```python
from build123d import *

# Parameters (mm, degrees)
BOSS_EXTRUDE1_DEPTH = 110


with BuildPart() as part:
    # Sketch1 → Boss-Extrude1 (new body)
    with BuildSketch(Plane.XY):
        Polygon((0, 12.5), (0, 0), (2, 0), (2, 9.5), (4, 9.5), (4, 0), (6, 0), (6, 9.5), (8, 9.5), (8, 0), (10, 0), (10, 9.5), (12, 9.5), (12, 0), (14, 0), (14, 9.5), (23.5, 9.5), (23.5, 12.5), align=None)
        Polygon((47, 12.5), (23.5, 12.5), (23.5, 9.5), (33, 9.5), (33, 0), (35, 0), (35, 9.5), (37, 9.5), (37, 0), (39, 0), (39, 9.5), (41, 9.5), (41, 0), (43, 0), (43, 9.5), (45, 9.5), (45, 0), (47, 0), align=None)
    extrude(amount=BOSS_EXTRUDE1_DEPTH)


solid = part.part
```
Geometry check sheet. Reference: the model listing, model coordinates, mm. A direction names the side the tool comes from. Coordinates: 2 decimals unless noted, no trailing zeros. Order: outer loops, then holes, each group sorted by start corner. A loop starts at its lowest first (then second) coordinate and runs counter-clockwise, first axis right, second up. Notation, with made-up numbers: M 34,-30 L 74,-30 A30 cw 74,-5 Z; hole C -0.5,7 d9. An arc over 180 degrees is marked long. Answer as a JSON object with one key per item and string values.
Q1. Tool access check on faces 1 (the flat face through (42, 0, 54)), 2 (the flat face through (45, 5, 54)). Record the directions out of +Z, -Z, +X, -X, +Y, -Y that give a thin tool (end or side, any length) a straight path to the whole face; none if there is none.
Results are:
{"face 1": "+Z, -Z, +X, -X, -Y", "face 2": "+Z, -Z, -Y"}
Q2. Scan line: line 1 (Y direction, x = 44, z = 38). Record every from-to range of solid material in increasing order.
Results are:
{"line 1": "y = 9.5 to 12.5"}
Q3. Cross-section at A-A on y = 8.25. Give the number of separate pieces and of enclosed holes in the cut face, and give its area (3 significant figures).
Results are:
{"separate pieces": "8", "enclosed holes": "0", "area": "1,760 mm²"}
Q4. Depth check by flat-ended pin: pin 1 Ø2 at (x, z) = (40.5, 46.5) entering from -Y; pin 2 Ø10 at (x, z) = (23, 86) entering from -Y. Enter the tip coordinate at first touch or a pass-through.
Results are:
{"pin 1": "stops at y = 0", "pin 2": "stops at y = 9.5"}
Q5. Cross-section at C-C on x = 28.5. Record the cut outline in (y, z).
Results are:
{"outline": "M 9.5,0 L 12.5,0 L 12.5,110 L 9.5,110 Z"}
Q6. Release check for a two-part mould opening along X. For faces 3 (the flat face through (47, 6, 54)), 4 (the flat face through (14, 5, 54)), 5 (the flat face through (9, 0, 54)) record: released by +X, released by -X, zero draft, split by the parting line, or undercut.
Results are:
{"face 3": "released by +X", "face 4": "undercut", "face 5": "zero draft"}
